Build history of the part. All positions in model axes, mm. Face numbers are marked on the shaded views. A direction names the side the tool comes from. Round coordinates to 2 decimals unless told otherwise and drop trailing zeros. Write each loop counter-clockwise with the first axis right and the second up, starting at its lowest first coordinate (ties: lowest second). Pieces come first, ordered by that corner, then holes. Notation, with made-up numbers: M 65.25,45 L 106.25,45 A25 ccw 106.25,74 Z; hole C -28.75,46.5 d8. An arc over 180 degrees is marked long. Use a Markdown table: item, result.
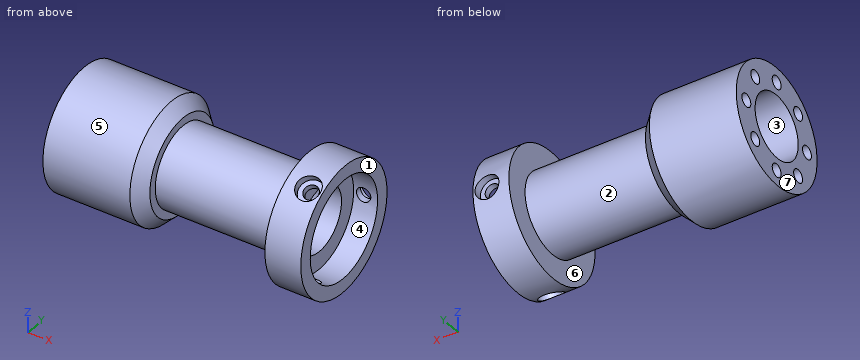
from build123d import *

# Parameters (mm, degrees)
SKETCH_2_R               = 8
CUT_EXTRUDE_1_DEPTH      = 70.156507286
SKETCH_5_R               = 12.5
CUT_EXTRUDE_2_DEPTH      = 6
CHAMFER_1_SIZE           = 3
PATTERN_CIRCULAR_3_COUNT = 8
PATTERN_CIRCULAR_4_COUNT = 3


# Read off the part's stored shape, not the designer's step: 打孔尺寸(%根据)内六角圆柱头螺钉的类型1
with BuildPart() as part:
    # 草图1 → 旋转1 (revolve)
    with BuildSketch(Plane(origin=(0, 0, 0), x_dir=(1, 0, 0), z_dir=(0, 1, 0)), mode=Mode.PRIVATE) as revolve_1_sk:
        Polygon((0, 0), (0, 15), (24.8, 15), (24.8, 10), (56.35, 10), (56.35, 16), (65.35, 16), (65.35, 0), align=None)
    revolve(revolve_1_sk.sketch.rotate(Axis((-27.673469388, 0, 0), (1, 0, 0)), 180), axis=Axis((-27.673469388, 0, 0), (1, 0, 0)))

    # 草图2 → 切除-拉伸1 (cut, through all)
    with BuildSketch(Plane.ZY):
        Circle(SKETCH_2_R)
    extrude(amount=-CUT_EXTRUDE_1_DEPTH, mode=Mode.SUBTRACT)

    # 草图5 → 切除-拉伸2 (cut)
    with BuildSketch(Plane(origin=(65.35, 0, 0), x_dir=(0, 0, -1), z_dir=(1, 0, 0))):
        Circle(SKETCH_5_R)
    extrude(amount=-CUT_EXTRUDE_2_DEPTH, mode=Mode.SUBTRACT)

    # 倒角1
    chamfer_1_edges = [part.edges().sort_by_distance(p)[0] for p in [
        (24.8, 0, -15),
    ]]
    chamfer(chamfer_1_edges, length=CHAMFER_1_SIZE)

    # 草图11 → M4 螺纹孔1 (revolve, cut)
    with BuildSketch(Plane.ZX.offset(11.25)):
        Polygon((0, 0), (0, 8.091420021), (1.65, 7.1), (1.65, 0), align=None)
    hole_wizard_m4_1 = revolve(axis=Axis((-6.35, 11.25, 0), (1, 0, 0)), mode=Mode.SUBTRACT)

    # 阵列(圆周)3: M4 螺纹孔1 ×8 about axis
    pattern_circular_3_axis = Axis((0, 0, 0), (1, 0, 0))
    for i in range(1, PATTERN_CIRCULAR_3_COUNT):
        add(hole_wizard_m4_1.rotate(pattern_circular_3_axis, i * 360 / PATTERN_CIRCULAR_3_COUNT), mode=Mode.SUBTRACT)

    # 打孔尺寸(%根据)内六角圆柱头螺钉的类型1 outline → 打孔尺寸(%根据)内六角圆柱头螺钉的类型1 (revolve, cut)
    with BuildSketch(Plane(origin=(61.85, 0, 0), x_dir=(1, 0, 0), z_dir=(0, 0, 1))):
        Polygon((1.8, 14), (3, 14), (3, 16.000041716), (0, 16.000041716), (0, 12.369650157), (1.8, 12.369650157), align=None)
    hole_wizard_1 = revolve(axis=Axis((61.85, 0, 0), (0, 1, 0)), mode=Mode.SUBTRACT)

    # 阵列(圆周)4: 打孔尺寸(%根据)内六角圆柱头螺钉的类型1 ×3 about axis
    pattern_circular_4_axis = Axis((0, 0, 0), (1, 0, 0))
    for i in range(1, PATTERN_CIRCULAR_4_COUNT):
        add(hole_wizard_1.rotate(pattern_circular_4_axis, i * 360 / PATTERN_CIRCULAR_4_COUNT), mode=Mode.SUBTRACT)


solid = part.part
Q1. Drop flat-ended pins along their axis: P1, Ø8, axis at x = 25.5, z = -11, coming from the -Y side; P2, Ø1, axis at x = 24.5, z = 11, coming from the +Y side; P3, Ø3, axis at y = 7.95, z = -7.95, coming from the -X side. Give the stop position or say it passes through.
Response values:
| item | result |
|---|---|
| P1 | stops at y = -11.71 |
| P2 | stops at y = 6.84 |
| P3 | stops at x = 7.19 |
Q2. Which spindle directions (+Z, -Z, +X, -X, +Y, -Y) get a long thin tool onto all of the face, cutting with end or side? Do the marked faces 4, 5, 6 and 7. Say none if no direction does.
Response values:
| item | result |
|---|---|
| face 4 | +X |
| face 5 | -X |
| face 6 | none |
| face 7 | +Z, -Z, -X, +Y, -Y |
Q3. Two-plate mould, pull along Z, no slides. Class the marked faces 1, 2 and 3: +Z half, -Z half, draft (parallel to the pull), parting line (faces both ways), or undercut.
Response values:
| item | result |
|---|---|
| face 1 | draft |
| face 2 | parting line |
| face 3 | undercut |
Q4. Cut at B-B on x = 21. Give the cut face in (y, z), and give its area (3 significant figures).
Response values:
| item | result |
|---|---|
| outline | C 0,0 d30; hole C 0,0 d16 |
| area | 506 mm2 |
Q5. Cut at A-A on x = 61.85. Give the cut face in (y, z).
Response values:
| item | result |
|---|---|
| outline | M -10.46,-12.11 L -9.6,-10.62 L -8.56,-11.22 L -7.74,-9.81 A12.5 cw -7.74,9.81 L -8.56,11.22 L -9.6,10.62 L -10.46,12.11 A16 ccw Z; M -5.44,-13.02 L -4.4,-13.62 L -5.26,-15.11 A16 ccw 15.72,-3 L 14,-3 L 14,-1.8 L 12.37,-1.8 A12.5 cw -4.63,-11.61 Z; M -5.44,13.02 L -4.63,11.61 A12.5 cw 12.37,1.8 L 14,1.8 L 14,3 L 15.72,3 A16 ccw -5.26,15.11 L -4.4,13.62 Z |
Q6. Drill centre lines: L1, parallel to X at y = 13, z = 0; L2, parallel to X at y = -3.5, z = -10; L3, parallel to Y at x = 7, z = 1.5. Where is each one in solid material? Low to high.
Response values:
| item | result |
|---|---|
| L1 | x = 0 to 23.8, 56.35 to 60.05, 63.65 to 65.35 |
| L2 | x = 0 to 24.8, 56.35 to 59.35 |
| L3 | y = -14.92 to -11.94, -10.56 to -7.86, 7.86 to 10.56, 11.94 to 14.92 |
Q7. Cut at D-D on x = 47.5. Give the cut face in (y, z), and give its area (3 significant figures).
Response values:
| item | result |
|---|---|
| outline | C 0,0 d20; hole C 0,0 d16 |
| area | 113 mm2 |
Q8. Cut at C-C on x = 6. Count the separate pieces of the cut face and the enclosed holes in it, and give its area (3 significant figures).
Response values:
| item | result |
|---|---|
| separate pieces | 1 |
| enclosed holes | 9 |
| area | 437 mm2 |
